```python
from build123d import *

# Parameters (mm, degrees)
BOSS_EXTRUDE1_DEPTH   = 1.5875
F_6_CLEARANCE_HOLE1_D = 4.3053


with BuildPart() as part:
    # Sketch1 → Boss-Extrude1 (new body)
    with BuildSketch(Plane.XY):
        Polygon((-41.367, 14.097), (6.663436815, 14.097), (23.618, 14.097), (23.618, -17.32), (92.658, -17.32), (92.658, 2.9845), (109.09675, 2.9845), (109.09675, -18.923), (99.008, -18.923), (92.658, -25.273), (92.658, -32.150898303), (109.09675, -32.150898303), (109.09675, -45.0855), (92.658, -45.0855), (92.658, -58.1655), (109.09675, -58.1655), (109.09675, -95.123), (90.082920323, -95.123), (9.878, -95.123), (-38.028966768, -95.123), (-58.86075, -95.123), (-58.86075, -58.1655), (-41.367, -58.1655), (-41.367, -45.0855), (-58.86075, -45.0855), (-58.86075, -13.0805), (-41.367, -13.0805), align=None)
    extrude(amount=BOSS_EXTRUDE1_DEPTH)

    # #6 Clearance Hole1 (through all)
    with Locations(Plane(origin=(0, 0, 0), x_dir=(-1, 0, 0), z_dir=(0, 0, -1))):
        with Locations((-106.398, -40.894), (-18.387, 10.287), (56.162, -40.894), (-18.387, -91.313)):
            Hole(F_6_CLEARANCE_HOLE1_D / 2)


solid = part.part
```
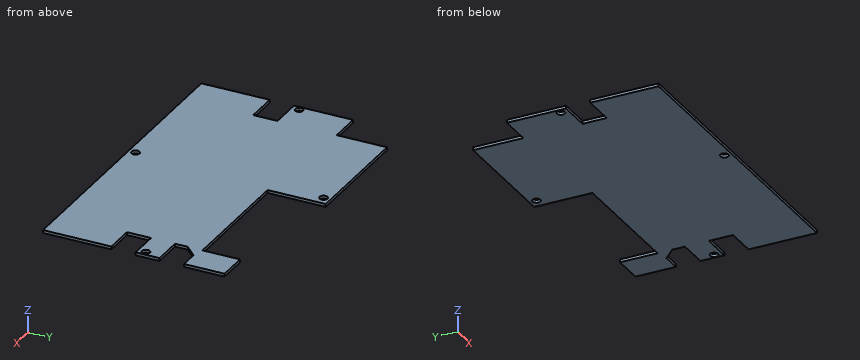
The model under review builds one solid part; all positions refer to its coordinate system, in mm. Round coordinates to 2 decimals unless told otherwise and drop trailing zeros. Loops run counter-clockwise (first coordinate to the right, second up) from the corner with the lowest first, then second, coordinate; pieces in that order, holes last. Notation, with made-up numbers: (-14, 65.25) -> (19, 65.25) arc R22 cw to (19, 102.25) -> close; hole circle Ø10 at (-38, 53). An arc over 180 degrees is marked (long way). Answer in a Markdown table with one row per item.
1) For pin 1 Ø0.8 at (y, z) = (-9.5, 0.5) entering from -X; pin 2 Ø0.8 at (x, z) = (98, 1) entering from +Y, all flat-tipped, find the tip position at first contact; note any pin that passes through.
Taken from the geometry:
| item | result |
|---|---|
| pin 1 | stops at x = -41.37 |
| pin 2 | stops at y = 2.98 |
2) Consider section C-C, the plane y = -54.5. Write out the cut boundary in (x, z).
Taken from the geometry:
| item | result |
|---|---|
| outline | (-41.37, 0) -> (92.66, 0) -> (92.66, 1.59) -> (-41.37, 1.59) -> close |
3) Consider section A-A, the plane y = -3. Write out the cut boundary in (x, z), plus the area to 3 significant figures.
Taken from the geometry:
| item | result |
|---|---|
| outline | (-41.37, 0) -> (23.62, 0) -> (23.62, 1.59) -> (-41.37, 1.59) -> close; (92.66, 0) -> (109.1, 0) -> (109.1, 1.59) -> (92.66, 1.59) -> close |
| area | 129 mm² |
4) Wall thickness on line 1 along X through (y, z) = (-4.5, 0.15); line 2 along Y through (x, z) = (94, 0.1); line 3 along Y through (x, z) = (96.5, 1.35): over which ranges is each line inside the solid? List them lowest first.
Taken from the geometry:
| item | result |
|---|---|
| line 1 | x = -41.37 to 23.62, 92.66 to 109.1 |
| line 2 | y = -95.12 to -58.17, -45.09 to -32.15, -23.93 to 2.98 |
| line 3 | y = -95.12 to -58.17, -45.09 to -32.15, -21.43 to 2.98 |
5) Consider section B-B, the plane z = 0.75. Write out the cut boundary in (x, y), plus the area to 3 significant figures.
Taken from the geometry:
| item | result |
|---|---|
| outline | (-58.86, -95.12) -> (109.1, -95.12) -> (109.1, -58.17) -> (92.66, -58.17) -> (92.66, -45.09) -> (109.1, -45.09) -> (109.1, -32.15) -> (92.66, -32.15) -> (92.66, -25.27) -> (99.01, -18.92) -> (109.1, -18.92) -> (109.1, 2.98) -> (92.66, 2.98) -> (92.66, -17.32) -> (23.62, -17.32) -> (23.62, 14.1) -> (-41.37, 14.1) -> (-41.37, -13.08) -> (-58.86, -13.08) -> (-58.86, -45.09) -> (-41.37, -45.09) -> (-41.37, -58.17) -> (-58.86, -58.17) -> close; hole circle Ø4.31 at (-56.16, -40.89); hole circle Ø4.31 at (18.39, -91.31); hole circle Ø4.31 at (18.39, 10.29); hole circle Ø4.31 at (106.4, -40.89) |
| area | 14,800 mm² |
6) Consider section D-D, the plane y = -22.5. Write out the cut boundary in (x, z), plus the area to 3 significant figures.
Taken from the geometry:
| item | result |
|---|---|
| outline | (-58.86, 0) -> (95.43, 0) -> (95.43, 1.59) -> (-58.86, 1.59) -> close |
| area | 245 mm² |
